```python
from build123d import *

# Parameters (mm, degrees)
COPYSKETCH010_W   = 200
COPYSKETCH010_H   = 130
COPYSKETCH010_R   = 1.75
COPYSKETCH010_R_2 = 3
COPYSKETCH010_R_3 = 6
COPYSKETCH010_W_2 = 15
COPYSKETCH010_H_2 = 15
PAD_DEPTH         = 3.5
PAD001_DEPTH      = 13.5
SKETCH001_R       = 0.75
POCKET_DEPTH      = 100
SKETCH002_R       = 0.75
POCKET001_DEPTH   = 5


with BuildPart() as part:
    # CopySketch010 → Pad (new body)
    with BuildSketch(Plane(origin=(0, 0, 0), x_dir=(-1, 0, 0), z_dir=(0, 0, -1))):
        with Locations((-100, 0)):
            Rectangle(COPYSKETCH010_W, COPYSKETCH010_H)
        with Locations((-196, 61)):
            Circle(COPYSKETCH010_R, mode=Mode.SUBTRACT)
        with Locations((-196, -61)):
            Circle(COPYSKETCH010_R, mode=Mode.SUBTRACT)
        with Locations((-125, -45)):
            Circle(COPYSKETCH010_R_2, mode=Mode.SUBTRACT)
        with Locations((-105, -45)):
            Circle(COPYSKETCH010_R_2, mode=Mode.SUBTRACT)
        with Locations((-85, -45)):
            Circle(COPYSKETCH010_R_2, mode=Mode.SUBTRACT)
        with Locations((-65, -45)):
            Circle(COPYSKETCH010_R_2, mode=Mode.SUBTRACT)
        with Locations((-50, -10)):
            Circle(COPYSKETCH010_R, mode=Mode.SUBTRACT)
        with Locations((-20, -10)):
            Circle(COPYSKETCH010_R, mode=Mode.SUBTRACT)
        with Locations((-50, 20)):
            Circle(COPYSKETCH010_R, mode=Mode.SUBTRACT)
        with Locations((-20, 20)):
            Circle(COPYSKETCH010_R, mode=Mode.SUBTRACT)
        with Locations((-160, -35)):
            Circle(COPYSKETCH010_R_3, mode=Mode.SUBTRACT)
        with Locations((-160, -5)):
            Circle(COPYSKETCH010_R_2, mode=Mode.SUBTRACT)
        with Locations((-35, -10)):
            Rectangle(COPYSKETCH010_W_2, COPYSKETCH010_H_2, mode=Mode.SUBTRACT)
        with Locations((-35, 20)):
            Rectangle(COPYSKETCH010_W_2, COPYSKETCH010_H_2, mode=Mode.SUBTRACT)
    extrude(amount=PAD_DEPTH)

    # Sketch → Pad001 (join)
    with BuildSketch(Plane.XY):
        Polygon((0, 65), (189, 65), (189, 62), (3, 62), (3, -62), (189, -62), (189, -65), (0, -65), align=None)
    extrude(amount=-PAD001_DEPTH)

    # Sketch001 → Pocket (cut, symmetric)
    with BuildSketch(Plane.XZ.offset(65)):
        with Locations((25, -8)):
            Circle(SKETCH001_R)
        with Locations((100, -8)):
            Circle(SKETCH001_R)
        with Locations((175, -8)):
            Circle(SKETCH001_R)
    extrude(amount=POCKET_DEPTH, both=True, mode=Mode.SUBTRACT)

    # Sketch002 → Pocket001 (cut)
    with BuildSketch(Plane.XZ.offset(-60)):
        with Locations((52, -7)):
            Circle(SKETCH002_R)
    extrude(amount=-POCKET001_DEPTH, mode=Mode.SUBTRACT)


solid = part.part
```
Input: part model. Units: mm. Frame: model coordinates. A direction names the side the tool comes from. Coordinates: 2 decimals unless noted, no trailing zeros. Write each loop counter-clockwise with the first axis right and the second up, starting at its lowest first coordinate (ties: lowest second). Pieces come first, ordered by that corner, then holes. Notation, with made-up numbers: (45.25, 8.25) -> (77.25, 8.25) arc R24 ccw to (77.25, 45.25) -> close; hole circle Ø5 at (15, 44.25). An arc over 180 degrees is marked (long way). Answer as a JSON object with one key per item and string values.
1. Section A-A on y = -35. Return the cut outline in (x, z), then the cut area to 3 significant figures.
Result set:
{"outline": "(0, -13.5) -> (3, -13.5) -> (3, -3.5) -> (154, -3.5) -> (154, 0) -> (0, 0) -> close; (166, -3.5) -> (200, -3.5) -> (200, 0) -> (166, 0) -> close", "area": "688 mm2"}
2. Mould query, pull axis X, two halves, no side actions, for faces 3 (the face through (0, -1, -7)), 4 (the face through (67.21, -42.97, -1.73)), 5 (the face through (97, 62, -8)). Classes: released by +X, released by -X, zero draft, split by the parting line, or undercut.
Result set:
{"face 3": "released by -X", "face 4": "undercut", "face 5": "zero draft"}
3. Section B-B on x = 29.5. Return the cut outline in (y, z), then the cut area to 3 significant figures.
Result set:
{"outline": "(-65, -13.5) -> (-62, -13.5) -> (-62, -3.5) -> (-17.5, -3.5) -> (-17.5, 0) -> (-65, 0) -> close; (-2.5, -3.5) -> (12.5, -3.5) -> (12.5, 0) -> (-2.5, 0) -> close; (27.5, -3.5) -> (62, -3.5) -> (62, -13.5) -> (65, -13.5) -> (65, 0) -> (27.5, 0) -> close", "area": "410 mm2"}
4. Material intervals for line 1 (Y direction, x = 160, z = -1.5); line 2 (Y direction, x = 196, z = -1.1); line 3 (Y direction, x = 97, z = -6.25), sorted ascending. Write a range as from..to.
Result set:
{"line 1": "y = -65..-41, -29..-8, -2..65", "line 2": "y = -65..-62.75, -59.25..59.25, 62.75..65", "line 3": "y = -65..-62, 62..65"}
5. Access query for faces 1 (the face through (3, 1, -8)), 2 (the face through (101, -65, -7)). Directions: +Z, -Z, +X, -X, +Y, -Y. A direction counts if a zero-diameter tool reaches every point of the face in a straight line with its end or side. Return the directions, or none.
Result set:
{"face 1": "-Z, +X", "face 2": "+Z, -Z, +X, -X, -Y"}
6. First-contact query: P1, Ø8, axis at x = 63, y = 20, coming from the -Z side; P2, Ø1.5, axis at y = 63, z = -8, coming from the +X side; P3, Ø5.5, axis at x = 125, y = -45, coming from the -Z side; P4, Ø8, axis at y = 20, z = -12, coming from the +X side. Flat tips, straight axial feed; report the tip coordinate or a pass-through.
Result set:
{"P1": "stops at z = -3.5", "P2": "stops at x = 189", "P3": "passes through", "P4": "stops at x = 3"}
7. Section D-D on x = 184.5. Return the cut outline in (y, z).
Result set:
{"outline": "(-65, -13.5) -> (-62, -13.5) -> (-62, -3.5) -> (62, -3.5) -> (62, -13.5) -> (65, -13.5) -> (65, 0) -> (-65, 0) -> close"}
8. Section C-C on x = 105. Return the cut outline in (y, z), then the cut area to 3 significant figures.
Result set:
{"outline": "(-65, -13.5) -> (-62, -13.5) -> (-62, -3.5) -> (-48, -3.5) -> (-48, 0) -> (-65, 0) -> close; (-42, -3.5) -> (62, -3.5) -> (62, -13.5) -> (65, -13.5) -> (65, 0) -> (-42, 0) -> close", "area": "494 mm2"}
